from build123d import *
from OCP.BRepFilletAPI import BRepFilletAPI_MakeChamfer

# Parameters (mm, degrees)
SKETCH1_W           = 107.95
SKETCH1_H           = 50.8
BOSS_EXTRUDE1_DEPTH = 3
SKETCH2_W           = 82.55
SKETCH2_H           = 50.8
SKETCH2_W_2         = 74.55
SKETCH2_H_2         = 42.8
BOSS_EXTRUDE2_DEPTH = 12
SKETCH3_R           = 5
SKETCH3_R_2         = 2.6
BOSS_EXTRUDE3_DEPTH = 5
CUT_EXTRUDE1_REACH  = 77.624
SKETCH4_W           = 55
SKETCH4_H           = 4
CUT_EXTRUDE2_REACH  = 101.713
SKETCH5_W           = 4
SKETCH5_H           = 20.8
SKETCH6_R           = 2.5
BOSS_EXTRUDE4_DEPTH = 12
CHAMFER1_SIZE       = 3
CHAMFER2_SIZE       = 3
CHAMFER2_SIZE_2     = 2.607860213
CHAMFER3_SIZE       = 1
CHAMFER3_SIZE2      = 1.191753593
SKETCH7_R           = 2.6
CUT_EXTRUDE3_DEPTH  = 6
CHAMFER4_SIZE       = 2
SKETCH8_R           = 2
CUT_EXTRUDE4_DEPTH  = 61.847848154
CHAMFER5_SIZE       = 5
FILLET1_R           = 3
CHAMFER6_SIZE       = 1
CHAMFER6_SIZE2      = 1.482560969


with BuildPart() as part:
    # Sketch1 → Boss-Extrude1 (new body)
    with BuildSketch(Plane.XY):
        Rectangle(SKETCH1_W, SKETCH1_H)
    extrude(amount=BOSS_EXTRUDE1_DEPTH)

    # Sketch2 → Boss-Extrude2 (add)
    with BuildSketch(Plane.XY.offset(3)):
        Rectangle(SKETCH2_W, SKETCH2_H)
        Rectangle(SKETCH2_W_2, SKETCH2_H_2, mode=Mode.SUBTRACT)
    extrude(amount=BOSS_EXTRUDE2_DEPTH)

    # Sketch3 → Boss-Extrude3 (add)
    # profile 1 of 4: a face of its own
    with BuildSketch(Plane.XY.offset(3)):
        with Locations((-23.275, 10.4)):
            Circle(SKETCH3_R)
        with Locations((-23.275, 10.4)):
            Circle(SKETCH3_R_2, mode=Mode.SUBTRACT)
    # profile 2 of 4: a face of its own
    with BuildSketch(Plane.XY.offset(3)):
        with Locations((-23.275, -9.823019498)):
            Circle(SKETCH3_R)
        with Locations((-23.275, -9.823019498)):
            Circle(SKETCH3_R_2, mode=Mode.SUBTRACT)
    # profile 3 of 4: a face of its own
    with BuildSketch(Plane.XY.offset(3)):
        with Locations((23.951190028, 10.4)):
            Circle(SKETCH3_R)
        with Locations((23.951190028, 10.4)):
            Circle(SKETCH3_R_2, mode=Mode.SUBTRACT)
    # profile 4 of 4: a face of its own
    with BuildSketch(Plane.XY.offset(3)):
        with Locations((23.951190028, -2.3)):
            Circle(SKETCH3_R)
        with Locations((23.951190028, -2.3)):
            Circle(SKETCH3_R_2, mode=Mode.SUBTRACT)
    extrude(amount=BOSS_EXTRUDE3_DEPTH)

    # Sketch4 → Cut-Extrude1 (cut, up to next)
    with BuildSketch(Plane.XZ.offset(25.4), mode=Mode.PRIVATE) as cut_extrude1_sk1:
        with Locations((-1.225, 13)):
            Rectangle(SKETCH4_W, SKETCH4_H)
    cut_extrude1_tool1 = extrude(cut_extrude1_sk1.sketch, amount=-CUT_EXTRUDE1_REACH, mode=Mode.PRIVATE) & part.part
    add(cut_extrude1_tool1.solids().sort_by_distance((-1.225, -25.4, 13))[0], mode=Mode.SUBTRACT)

    # Sketch5 → Cut-Extrude2 (cut, up to next)
    with BuildSketch(Plane.ZY.offset(41.275), mode=Mode.PRIVATE) as cut_extrude2_sk1:
        with Locations((13, 0)):
            Rectangle(SKETCH5_W, SKETCH5_H)
    cut_extrude2_tool1 = extrude(cut_extrude2_sk1.sketch, amount=-CUT_EXTRUDE2_REACH, mode=Mode.PRIVATE) & part.part
    add(cut_extrude2_tool1.solids().sort_by_distance((-41.275, 0, 13))[0], mode=Mode.SUBTRACT)

    # Sketch6 → Boss-Extrude4 (add)
    with BuildSketch(Plane.XY.offset(15)):
        with BuildLine():
            Line((-33.275, 12.9), (-28.775, 17.4))
            Line((-28.775, 17.4), (-28.775, 21.4))
            Line((-28.775, 21.4), (-33.983712153, 21.4))
            ThreePointArc((-33.983712153, 21.4), (-33.827734218, 20.910774109), (-33.775, 20.4))
            ThreePointArc((-33.775, 20.4), (-34.905693606, 18.308349934), (-37.275, 18.108712153))
            Line((-37.275, 18.108712153), (-37.275, 12.9))
            Line((-37.275, 12.9), (-33.275, 12.9))
        make_face()
        with Locations((-36.275, -20.4)):
            Circle(SKETCH6_R)
        Polygon((-37.275, -12.9), (-37.275, -21.4), (-28.775, -21.4), (-28.775, -17.4), (-33.275, -12.9), align=None)
        with BuildLine():
            Line((37.275, -18.108712153), (37.275, -12.9))
            Line((37.275, -12.9), (33.275, -12.9))
            Line((33.275, -12.9), (28.775, -17.4))
            Line((28.775, -17.4), (28.775, -21.4))
            Line((28.775, -21.4), (33.983712153, -21.4))
            ThreePointArc((33.983712153, -21.4), (34.507233047, -18.632233047), (37.275, -18.108712153))
        make_face()
        with BuildLine():
            Line((33.983712153, 21.4), (28.775, 21.4))
            Line((28.775, 21.4), (28.775, 17.4))
            Line((28.775, 17.4), (33.275, 12.9))
            Line((33.275, 12.9), (37.275, 12.9))
            Line((37.275, 12.9), (37.275, 18.108712153))
            ThreePointArc((37.275, 18.108712153), (34.507233047, 18.632233047), (33.983712153, 21.4))
        make_face()
        with BuildLine():
            ThreePointArc((-33.775, 20.4), (-33.827734218, 20.910774109), (-33.983712153, 21.4))
            Line((-33.983712153, 21.4), (-37.275, 21.4))
            Line((-37.275, 21.4), (-37.275, 18.108712153))
            ThreePointArc((-37.275, 18.108712153), (-34.905693606, 18.308349934), (-33.775, 20.4))
        make_face()
        with BuildLine():
            Line((-37.275, 21.4), (-33.983712153, 21.4))
            ThreePointArc((-33.983712153, 21.4), (-38.042766953, 22.167766953), (-37.275, 18.108712153))
            Line((-37.275, 18.108712153), (-37.275, 21.4))
        make_face()
        with BuildLine():
            ThreePointArc((-37.275, -18.108712153), (-38.042766953, -22.167766953), (-33.983712153, -21.4))
            Line((-33.983712153, -21.4), (-37.275, -21.4))
            Line((-37.275, -21.4), (-37.275, -18.108712153))
        make_face()
        with BuildLine():
            Line((-37.275, -21.4), (-33.983712153, -21.4))
            ThreePointArc((-33.983712153, -21.4), (-33.827734218, -20.910774109), (-33.775, -20.4))
            ThreePointArc((-33.775, -20.4), (-34.905693606, -18.308349934), (-37.275, -18.108712153))
            Line((-37.275, -18.108712153), (-37.275, -21.4))
        make_face()
        with BuildLine():
            ThreePointArc((38.775, 20.4), (36.785774109, 22.847265782), (33.983712153, 21.4))
            Line((33.983712153, 21.4), (37.275, 21.4))
            Line((37.275, 21.4), (37.275, 18.108712153))
            ThreePointArc((37.275, 18.108712153), (38.366650066, 19.030693606), (38.775, 20.4))
        make_face()
        with BuildLine():
            Line((37.275, 21.4), (33.983712153, 21.4))
            ThreePointArc((33.983712153, 21.4), (34.507233047, 18.632233047), (37.275, 18.108712153))
            Line((37.275, 18.108712153), (37.275, 21.4))
        make_face()
        with BuildLine():
            ThreePointArc((38.775, -20.4), (38.366650066, -19.030693606), (37.275, -18.108712153))
            Line((37.275, -18.108712153), (37.275, -21.4))
            Line((37.275, -21.4), (33.983712153, -21.4))
            ThreePointArc((33.983712153, -21.4), (36.785774109, -22.847265782), (38.775, -20.4))
        make_face()
        with BuildLine():
            Line((37.275, -21.4), (37.275, -18.108712153))
            ThreePointArc((37.275, -18.108712153), (34.507233047, -18.632233047), (33.983712153, -21.4))
            Line((33.983712153, -21.4), (37.275, -21.4))
        make_face()
    extrude(amount=-BOSS_EXTRUDE4_DEPTH)

    # Chamfer1
    chamfer1_edges = [part.edges().sort_by_distance(p)[0] for p in [
        (-41.275, 25.4, 9),
        (-41.275, -25.4, 9),
        (41.275, -25.4, 9),
        (41.275, 25.4, 9),
    ]]
    chamfer(chamfer1_edges, length=CHAMFER1_SIZE)

    # Chamfer2
    # the kernel refuses this chamfer: 3, 2.607860213 mm, written as the material it adds along each edge
    with BuildSketch(Plane(origin=(-23.275, 10.4, 3), x_dir=(1, 0, 0), z_dir=(0, -1, 0))) as chamfer2_piece_1:
        Polygon((5 + CHAMFER2_SIZE, 0), (5, CHAMFER2_SIZE_2), (5, 0), align=None)
    revolve(axis=Axis((-23.275, 10.4, 3), (0, 0, 1)))
    with BuildSketch(Plane(origin=(-23.275, -9.823019498, 3), x_dir=(1, 0, 0), z_dir=(0, -1, 0))) as chamfer2_piece_2:
        Polygon((5 + CHAMFER2_SIZE, 0), (5, CHAMFER2_SIZE_2), (5, 0), align=None)
    revolve(axis=Axis((-23.275, -9.823019498, 3), (0, 0, 1)))
    with BuildSketch(Plane(origin=(23.951190028, 10.4, 3), x_dir=(1, 0, 0), z_dir=(0, -1, 0))) as chamfer2_piece_3:
        Polygon((5 + CHAMFER2_SIZE, 0), (5, CHAMFER2_SIZE_2), (5, 0), align=None)
    revolve(axis=Axis((23.951190028, 10.4, 3), (0, 0, 1)))
    with BuildSketch(Plane(origin=(23.951190028, -2.3, 3), x_dir=(1, 0, 0), z_dir=(0, -1, 0))) as chamfer2_piece_4:
        Polygon((5 + CHAMFER2_SIZE, 0), (5, CHAMFER2_SIZE_2), (5, 0), align=None)
    revolve(axis=Axis((23.951190028, -2.3, 3), (0, 0, 1)))

    # Chamfer3: one chamfer whose edges measure the first distance from different faces: ONE call of the kernel's chamfer builder (chamfer() names one face for all edges)
    chamfer3_edges_1 = [part.edges().sort_by_distance(p)[0] for p in [
        (-25.875, 10.4, 8),
    ]]
    chamfer3_side_1 = [part.faces().sort_by_distance(p)[0] for p in [
        (-28.133578644, 10.4, 8),
    ]]
    chamfer3_edges_2 = [part.edges().sort_by_distance(p)[0] for p in [
        (-25.875, -9.823019498, 8),
    ]]
    chamfer3_side_2 = [part.faces().sort_by_distance(p)[0] for p in [
        (-28.133578644, -9.823019498, 8),
    ]]
    chamfer3_edges_3 = [part.edges().sort_by_distance(p)[0] for p in [
        (21.351190028, 10.4, 8),
    ]]
    chamfer3_side_3 = [part.faces().sort_by_distance(p)[0] for p in [
        (19.092611384, 10.4, 8),
    ]]
    chamfer3_edges_4 = [part.edges().sort_by_distance(p)[0] for p in [
        (21.351190028, -2.3, 8),
    ]]
    chamfer3_side_4 = [part.faces().sort_by_distance(p)[0] for p in [
        (19.092611384, -2.3, 8),
    ]]
    chamfer3 = BRepFilletAPI_MakeChamfer(part.part.solid().wrapped)
    for e in chamfer3_edges_1:
        chamfer3.Add(CHAMFER3_SIZE, CHAMFER3_SIZE2, e.wrapped, chamfer3_side_1[0].wrapped)  # the first distance lies on this face
    for e in chamfer3_edges_2:
        chamfer3.Add(CHAMFER3_SIZE, CHAMFER3_SIZE2, e.wrapped, chamfer3_side_2[0].wrapped)  # the first distance lies on this face
    for e in chamfer3_edges_3:
        chamfer3.Add(CHAMFER3_SIZE, CHAMFER3_SIZE2, e.wrapped, chamfer3_side_3[0].wrapped)  # the first distance lies on this face
    for e in chamfer3_edges_4:
        chamfer3.Add(CHAMFER3_SIZE, CHAMFER3_SIZE2, e.wrapped, chamfer3_side_4[0].wrapped)  # the first distance lies on this face
    add(Compound.cast(chamfer3.Shape()), mode=Mode.REPLACE)

    # Sketch7 → Cut-Extrude3 (cut)
    with BuildSketch(Plane.XY.offset(15)):
        with Locations((-36.275, 20.4)):
            Circle(SKETCH7_R)
        with Locations((-36.275, -20.4)):
            Circle(SKETCH7_R)
        with Locations((36.275, 20.4)):
            Circle(SKETCH7_R)
        with Locations((36.275, -20.4)):
            Circle(SKETCH7_R)
    extrude(amount=-CUT_EXTRUDE3_DEPTH, mode=Mode.SUBTRACT)

    # Chamfer4
    chamfer4_edges = [part.edges().sort_by_distance(p)[0] for p in [
        (26.275, -23.4, 11),
        (-28.725, -23.4, 11),
        (-39.275, 10.4, 11),
        (-39.275, -10.4, 11),
    ]]
    chamfer(chamfer4_edges, length=CHAMFER4_SIZE)

    # Sketch8 → Cut-Extrude4 (cut, through all)
    with BuildSketch(Plane.XY.offset(3)):
        with Locations((-47.625, 19.05)):
            Circle(SKETCH8_R)
        with Locations((-47.625, -19.05)):
            Circle(SKETCH8_R)
        with Locations((47.625, 19.05)):
            Circle(SKETCH8_R)
        with Locations((47.625, -19.05)):
            Circle(SKETCH8_R)
    extrude(amount=-CUT_EXTRUDE4_DEPTH, mode=Mode.SUBTRACT)

    # Chamfer5
    chamfer5_edges = [part.edges().sort_by_distance(p)[0] for p in [
        (-53.975, 25.4, 1.5),
        (53.975, 25.4, 1.5),
        (53.975, -25.4, 1.5),
        (-53.975, -25.4, 1.5),
    ]]
    chamfer(chamfer5_edges, length=CHAMFER5_SIZE)

    # Fillet1
    fillet1_edges = [part.edges().sort_by_distance(p)[0] for p in [
        (-41.275, 0, 3),
        (41.275, 0, 3),
        (-39.775, 23.9, 3),
        (39.775, 23.9, 3),
        (39.775, -23.9, 3),
        (-39.775, -23.9, 3),
    ]]
    fillet(fillet1_edges, radius=FILLET1_R)

    # Chamfer6: one chamfer whose edges measure the first distance from different faces: ONE call of the kernel's chamfer builder (chamfer() names one face for all edges)
    chamfer6_edges_1 = [part.edges().sort_by_distance(p)[0] for p in [
        (-38.875, -20.4, 15),
    ]]
    chamfer6_side_1 = [part.faces().sort_by_distance(p)[0] for p in [
        (-38.875, -20.4, 12),
    ]]
    chamfer6_edges_2 = [part.edges().sort_by_distance(p)[0] for p in [
        (33.675, 20.4, 15),
    ]]
    chamfer6_side_2 = [part.faces().sort_by_distance(p)[0] for p in [
        (33.675, 20.4, 12),
    ]]
    chamfer6_edges_3 = [part.edges().sort_by_distance(p)[0] for p in [
        (33.675, -20.4, 15),
        (-38.875, 20.4, 15),
    ]]
    chamfer6_side_3 = [part.faces().sort_by_distance(p)[0] for p in [
        (-40.305714567, 16.4, 15),
    ]]
    chamfer6 = BRepFilletAPI_MakeChamfer(part.part.solid().wrapped)
    for e in chamfer6_edges_1:
        chamfer6.Add(CHAMFER6_SIZE, CHAMFER6_SIZE2, e.wrapped, chamfer6_side_1[0].wrapped)  # the first distance lies on this face
    for e in chamfer6_edges_2:
        chamfer6.Add(CHAMFER6_SIZE, CHAMFER6_SIZE2, e.wrapped, chamfer6_side_2[0].wrapped)  # the first distance lies on this face
    for e in chamfer6_edges_3:
        chamfer6.Add(CHAMFER6_SIZE, CHAMFER6_SIZE2, e.wrapped, chamfer6_side_3[0].wrapped)  # the first distance lies on this face
    add(Compound.cast(chamfer6.Shape()), mode=Mode.REPLACE)


solid = part.part
Here's how the part is built. I have some questions about the finished solid (model axes, mm). A direction names the side the tool comes from. Round coordinates to 2 decimals unless told otherwise and drop trailing zeros. Loops run counter-clockwise (first coordinate to the right, second up) from the corner with the lowest first, then second, coordinate; pieces in that order, holes last. Notation, with made-up numbers: (-2, -34.75) -> (52, -34.75) arc R13 cw to (52, -20.75) -> close; hole circle Ø5 at (4, 82). An arc over 180 degrees is marked (long way). Write each question's results on one line, items separated by ' | '.
(1) We'd pull the mould along Y, two halves only. Please class faces 1 (the face through (-35, -12.9, 9)), 2 (the face through (-23, -10, 3)), 3 (the face through (-51.51, -22.865, 1.479)), 4 (the face through (-53.975, 0, 1)): released by +Y, released by -Y, zero draft, split by the parting line, or undercut.
Worked answers:
face 1: undercut | face 2: undercut | face 3: released by -Y | face 4: zero draft
(2) For faces 5 (the face through (26.275, -23, 14)), 6 (the face through (-41.275, 0, 9)), 7 (the face through (28.775, -19, 9)), 8 (the face through (-39, 10.4, 14)), which set-ups out of +Z, -Z, +X, -X, +Y, -Y let a thin tool reach every point of the face, with its end or its side?
Worked answers:
face 5: +Z, -Y | face 6: +Z, -X, +Y, -Y | face 7: +Z | face 8: +Z, -X
(3) If we section it at B-B, the plane x = -1: List the corners of the cut face in (y, z) for me.
Worked answers:
outline: (-25.4, 0) -> (25.4, 0) -> (25.4, 15) -> (21.4, 15) -> (21.4, 3) -> (-21.4, 3) -> (-21.4, 11) -> (-25.4, 11) -> close
(4) If we section it at A-A, the plane z = 1: List the corners of the cut face in (x, y) for me (3 decimals).
Worked answers:
outline: (-53.975, -20.4) -> (-48.975, -25.4) -> (48.975, -25.4) -> (53.975, -20.4) -> (53.975, 20.4) -> (48.975, 25.4) -> (-48.975, 25.4) -> (-53.975, 20.4) -> close; hole circle Ø4 at (-47.625, -19.05); hole circle Ø4 at (-47.625, 19.05); hole circle Ø4 at (47.625, -19.05); hole circle Ø4 at (47.625, 19.05)
(5) For P1, Ø1.2, axis at y = -18.5, z = 11.5, coming from the +X side (3 decimals); P2, Ø0.6, axis at x = -39, z = 14, coming from the +Y side (3 decimals); P3, Ø3, axis at x = -39, y = -1, coming from the +Z side, each with a flat end and sliding along its axis, tell me the tip position at first contact or that it passes through.
Worked answers:
P1: x = 41.275 | P2: y = 24.975 | P3: z = 11
(6) If I drill on L1, parallel to Y at x = -15, z = 10.5; L2, parallel to Y at x = -33.5, z = 7.5; L3, parallel to X at y = 20, z = 6.5 (3 decimals), over which ranges is the centre line in solid material (lowest first)?
Worked answers:
L1: -25.4 to -21.4, 21.4 to 25.4 | L2: -25.4 to -12.9, 12.9 to 25.4 | L3: -41.275 to -28.775, 28.775 to 41.275
